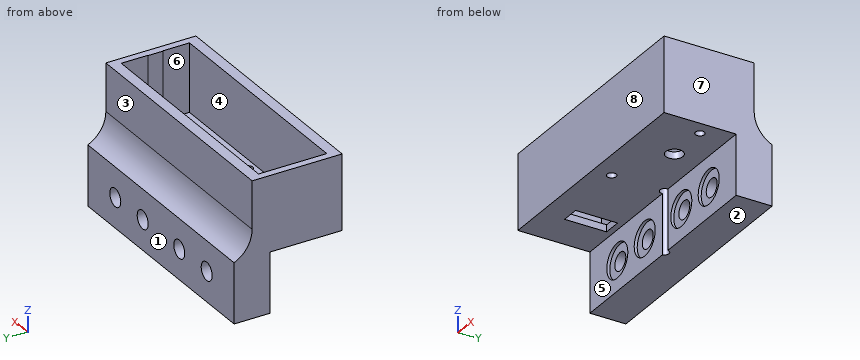
```python
from build123d import *

# Parameters (mm, degrees)
SKETCH1_W                 = 80
SKETCH1_H                 = 30
MOTOR_HOUSING_DEPTH       = 25
SKETCH2_W                 = 80
SKETCH2_H                 = 6
ATATACH_TO_BODY_R_DEPTH   = 20
FILLET_R_R                = 10
SCREW_START               = -12
SKETCH3_R                 = 5.75
SKETCH3_R_2               = 3
SCREW_HEAD_INSETS_R_DEPTH = 1
SKETCH3_2_R               = 3
SCREW_HOLES_R_DEPTH       = 74.569203879
SKETCH4_R                 = 1.5
SKETCH4_R_2               = 2.85
SKETCH4_W                 = 6
SKETCH4_H                 = 14
MOTOR_HOLES_DEPTH         = 96.407286673
SKETCH4_3_R               = 1.5
SKETCH4_3_R_2             = 2.85
SKETCH4_3_W               = 6
SKETCH4_3_H               = 14
MOTOR_CAVITY_DEPTH        = 22.7
SKETCH4_4_W               = 4.8
SKETCH4_4_H               = 5
SKETCH4_4_R               = 1.5
MOUNT_STABILITY_DEPTH     = 16.7


with BuildPart() as part:
    # Sketch1 → Motor Housing (new body)
    with BuildSketch(Plane.XY):
        with Locations((-19.08830476, 38.88424326)):
            Rectangle(SKETCH1_W, SKETCH1_H)
    extrude(amount=MOTOR_HOUSING_DEPTH)

    # Sketch2 → Atatach to Body R (add)
    with BuildSketch(Plane(origin=(0, 0, 0), x_dir=(-1, 0, 0), z_dir=(0, 0, -1))):
        with Locations((19.08830476, 50.88424326)):
            Rectangle(SKETCH2_W, SKETCH2_H)
        with Locations((19.08830476, 56.88424326)):
            Rectangle(SKETCH2_W, SKETCH2_H)
    extrude(amount=ATATACH_TO_BODY_R_DEPTH)

    # Fillet R
    # the kernel refuses this fillet: 10 mm, written as the material it adds along each edge
    with BuildSketch(Plane(origin=(-59.08830476, 53.88424326, 0), x_dir=(0, 0, 1), z_dir=(1, 0, 0))) as fillet_r_piece_1:
        with BuildLine():
            CenterArc((9.16515139, -10), FILLET_R_R, 90, 66.421821522)
            Line((0, -6), (-0.183303028, -5.92))
            ThreePointArc((-0.183303028, -5.92), (-0.2, -3), (-0.2, 0))
            Line((-0.2, 0), (0, 0.2))
            Line((0, 0.2), (9.16515139, 0.2))
            Line((9.16515139, 0.2), (9.16515139, 0))
        make_face()
    extrude(amount=80)

    # Sketch3 → Screw Head Insets R (cut)
    # profile 1 of 4: a face of its own
    with BuildSketch(Plane(origin=(0, 59.88424326, 0), x_dir=(1, 0, 0), z_dir=(0, 1, 0)).offset(SCREW_START)):
        with Locations(Location((-44.08830476, 10, 0), (0, 0, 270))):
            Circle(SKETCH3_R)
        with Locations(Location((-44.08830476, 10, 0), (0, 0, 270))):
            Circle(SKETCH3_R_2, mode=Mode.SUBTRACT)
    # profile 2 of 4: a face of its own
    with BuildSketch(Plane(origin=(0, 59.88424326, 0), x_dir=(1, 0, 0), z_dir=(0, 1, 0)).offset(SCREW_START)):
        with Locations(Location((-29.08830476, 10, 0), (0, 0, 270))):
            Circle(SKETCH3_R)
        with Locations(Location((-29.08830476, 10, 0), (0, 0, 270))):
            Circle(SKETCH3_R_2, mode=Mode.SUBTRACT)
    # profile 3 of 4: a face of its own
    with BuildSketch(Plane(origin=(0, 59.88424326, 0), x_dir=(1, 0, 0), z_dir=(0, 1, 0)).offset(SCREW_START)):
        with Locations(Location((5.91169524, 10, 0), (0, 0, 270))):
            Circle(SKETCH3_R)
        with Locations(Location((5.91169524, 10, 0), (0, 0, 270))):
            Circle(SKETCH3_R_2, mode=Mode.SUBTRACT)
    # profile 4 of 4: a face of its own
    with BuildSketch(Plane(origin=(0, 59.88424326, 0), x_dir=(1, 0, 0), z_dir=(0, 1, 0)).offset(SCREW_START)):
        with Locations(Location((-9.08830476, 10, 0), (0, 0, 270))):
            Circle(SKETCH3_R)
        with Locations(Location((-9.08830476, 10, 0), (0, 0, 270))):
            Circle(SKETCH3_R_2, mode=Mode.SUBTRACT)
    extrude(amount=SCREW_HEAD_INSETS_R_DEPTH, mode=Mode.SUBTRACT)

    # Sketch3<2> → Screw Holes R (cut, through all)
    with BuildSketch(Plane(origin=(0, 59.88424326, 0), x_dir=(1, 0, 0), z_dir=(0, 1, 0))):
        with Locations(Location((5.91169524, 10, 0), (0, 0, 270))):
            Circle(SKETCH3_2_R)
        with Locations(Location((-9.08830476, 10, 0), (0, 0, 270))):
            Circle(SKETCH3_2_R)
        with Locations(Location((-29.08830476, 10, 0), (0, 0, 270))):
            Circle(SKETCH3_2_R)
        with Locations(Location((-44.08830476, 10, 0), (0, 0, 270))):
            Circle(SKETCH3_2_R)
    extrude(amount=-SCREW_HOLES_R_DEPTH, mode=Mode.SUBTRACT)

    # Sketch4 → Motor Holes (cut, through all)
    with BuildSketch(Plane.XY.offset(25)):
        with Locations((-17.93830476, 47.68424326)):
            Circle(SKETCH4_R)
        with Locations((-17.93830476, 30.08424326)):
            Circle(SKETCH4_R)
        with Locations((1.91169524, 38.88424326)):
            Circle(SKETCH4_R_2)
        with Locations((15.91169524, 38.88424326)):
            Circle(SKETCH4_R)
        with Locations((-43.63830476, 38.88424326)):
            Rectangle(SKETCH4_W, SKETCH4_H)
    extrude(amount=-MOTOR_HOLES_DEPTH, mode=Mode.SUBTRACT)

    # Sketch4<3> → Motor Cavity (cut)
    with BuildSketch(Plane.XY.offset(25)):
        Polygon((18.46169524, 50.25424326), (-56.63830476, 50.25424326), (-56.63830476, 27.51424326), (18.46169524, 27.51424326), (18.46169524, 36.38424326), (18.31169524, 36.38424326), (13.51169524, 36.38424326), (13.51169524, 41.38424326), (18.31169524, 41.38424326), (18.46169524, 41.38424326), align=None)
        with Locations((-17.93830476, 30.08424326)):
            Circle(SKETCH4_3_R, mode=Mode.SUBTRACT)
        with Locations((1.91169524, 38.88424326)):
            Circle(SKETCH4_3_R_2, mode=Mode.SUBTRACT)
        with Locations((-43.63830476, 38.88424326)):
            Rectangle(SKETCH4_3_W, SKETCH4_3_H, mode=Mode.SUBTRACT)
        with Locations((-17.93830476, 47.68424326)):
            Circle(SKETCH4_3_R, mode=Mode.SUBTRACT)
    extrude(amount=-MOTOR_CAVITY_DEPTH, mode=Mode.SUBTRACT)

    # Sketch4<4> → Mount Stability (cut)
    with BuildSketch(Plane.XY.offset(25)):
        with Locations((15.91169524, 38.88424326)):
            Rectangle(SKETCH4_4_W, SKETCH4_4_H)
        with Locations((15.91169524, 38.88424326)):
            Circle(SKETCH4_4_R, mode=Mode.SUBTRACT)
    extrude(amount=-MOUNT_STABILITY_DEPTH, mode=Mode.SUBTRACT)


solid = part.part
```
The model under review builds one solid part; all positions refer to its coordinate system, in mm. Face numbers are marked on the shaded views. A direction names the side the tool comes from. Round coordinates to 2 decimals unless told otherwise and drop trailing zeros. Loops run counter-clockwise (first coordinate to the right, second up) from the corner with the lowest first, then second, coordinate; pieces in that order, holes last.
Item 1: Mouldability with a two-part tool opening along X and no side actions: class the marked faces 6, 7 and 8 as released by +X, released by -X, zero draft, split by the parting line, or undercut.
Determined:
face 6: undercut
face 7: released by +X
face 8: zero draft
Item 2: Take a section at B-B (z = 14.5). Write out the cut boundary in (x, y).
Determined:
outline: (-59.09, 23.88) - (20.91, 23.88) - (20.91, 53.88) - (-59.09, 53.88) - close; hole (-56.64, 27.51) - (18.46, 27.51) - (18.46, 36.38) - (18.31, 36.38) - (18.31, 41.38) - (18.46, 41.38) - (18.46, 50.25) - (-56.64, 50.25) - close
Item 3: For line 1 (X direction, y = 57, z = -10); line 2 (X direction, y = 31.5, z = 15.5); line 3 (Y direction, x = 17, z = 3), list the stretches that pass through material, from the lowest coordinate up.
Determined:
line 1: x = -59.09 to -47.09, -41.09 to -32.09, -26.09 to -12.09, -6.09 to 2.91, 8.91 to 20.91
line 2: x = -59.09 to -56.64, 18.46 to 20.91
line 3: y = 23.88 to 27.51, 36.38 to 37.85, 39.92 to 41.38, 50.25 to 56.01
Item 4: Take a section at D-D (z = 3.5). Write out the cut boundary in (x, y), then the cut area to 3 significant figures.
Determined:
outline: (-59.09, 23.88) - (20.91, 23.88) - (20.91, 55.64) - (-59.09, 55.64) - close; hole (-56.64, 27.51) - (18.46, 27.51) - (18.46, 36.38) - (13.51, 36.38) - (13.51, 41.38) - (18.46, 41.38) - (18.46, 50.25) - (-56.64, 50.25) - close; hole circle Ø3 at (15.91, 38.88)
area: 851 mm2
Item 5: For the marked faces 1, 2, 3, 4 and 5, list the 3-axis set-ups (+Z, -Z, +X, -X, +Y, -Y) from which the entire face can be reached by the end or side of a thin tool; tool diameter is ignored.
Determined:
face 1: +Z, -Z, +X, -X, +Y
face 2: -Z, +X, -X, +Y, -Y
face 3: +Z, +X, -X, +Y
face 4: +Z
face 5: -Z, +X, -X, -Y
Item 6: Take a section at C-C (x = -30). Write out the cut boundary in (y, z).
Determined:
outline: (23.88, 0) - (47.88, 0) - (47.88, -4.32) - (48.88, -4.32) - (48.88, -7.14) - (59.88, -7.14) - (59.88, 0) arc R10 cw to (53.88, 9.17) - (53.88, 25) - (50.25, 25) - (50.25, 2.3) - (27.51, 2.3) - (27.51, 25) - (23.88, 25) - close; (47.88, -20) - (59.88, -20) - (59.88, -12.86) - (48.88, -12.86) - (48.88, -15.68) - (47.88, -15.68) - close
Item 7: Take a section at A-A (y = 34.5). Write out the cut boundary in (x, z), then the cut area to 3 significant figures.
Determined:
outline: (-59.09, 0) - (-46.64, 0) - (-46.64, 2.3) - (-56.64, 2.3) - (-56.64, 25) - (-59.09, 25) - close; (-40.64, 0) - (20.91, 0) - (20.91, 25) - (18.46, 25) - (18.46, 2.3) - (-40.64, 2.3) - close
area: 281 mm2
Item 8: Clearance check with flat-ended pins moving along their axes: pin 1 Ø3.5 at (x, y) = (-17.94, 30.08) entering from -Z; pin 2 Ø4 at (x, y) = (-16.5, 47.5) entering from +Z; pin 3 Ø18.5 at (x, z) = (-29.09, -10) entering from +Y; pin 4 Ø12.5 at (x, z) = (-5.5, 15.5) entering from +Y. State where each tip first meets the part, or that it passes through.
Determined:
pin 1: stops at z = 0
pin 2: stops at z = 2.3
pin 3: stops at y = 59.88
pin 4: stops at y = 53.88
